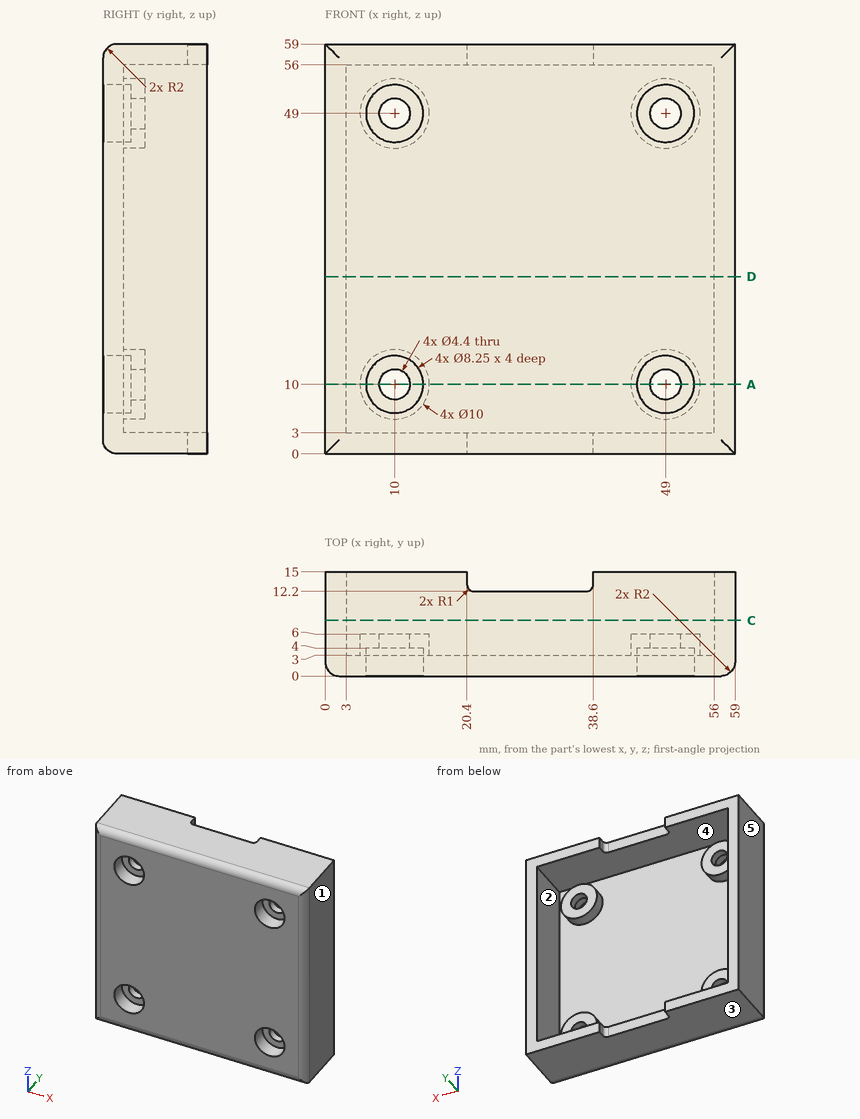
Can you work these out from the drawing? Everything is in mm from the part's minimum corner. A direction names the side the tool comes from. Round coordinates to 2 decimals unless told otherwise and drop trailing zeros. Order: outer loops, then holes, each group sorted by start corner. A loop starts at its lowest first (then second) coordinate and runs counter-clockwise, first axis right, second up. Notation, with made-up numbers: M 86,-9.5 L 132,-9.5 A20 ccw 132,5.5 Z; hole C -1,25 d11. An arc over 180 degrees is marked long. One line per question, with ' | ' between items.
1) For the marked faces 1 and 2, which set-ups out of +Z, -Z, +X, -X, +Y, -Y let a thin tool reach every point of the face, with its end or its side?
Working result:
face 1: +Z, -Z, +X, +Y, -Y | face 2: +Y
2) If we mould it in two halves opening along Z, with no side actions, what happens to the marked faces 3, 4 and 5? For each: +Z half, -Z half, draft (parallel to the pull), parting line (faces both ways), or undercut.
Working result:
face 3: -Z half | face 4: undercut | face 5: draft
3) I want a section at D-D, the plane z = 25.5. Write out the boundary of the cut face in (x, y), then the cut area to 3 significant figures.
Working result:
outline: M 0,2 A2 ccw 2,0 L 57,0 A2 ccw 59,2 L 59,15 L 56,15 L 56,3 L 3,3 L 3,15 L 0,15 Z | area: 247 mm²
4) I want a section at C-C, the plane y = 8. Write out the boundary of the cut face in (x, z).
Working result:
outline: M 0,0 L 59,0 L 59,59 L 0,59 Z; hole M 3,3 L 56,3 L 56,56 L 3,56 Z
5) I need wall thicknesses on line 1 along Z through (x, y) = (49, 5.3); line 2 along Z through (x, y) = (42, 14); line 3 along Z through (x, y) = (49, 2.3) (3 decimals). Which ranges of each line are inside material? Lowest first, please.
Working result:
line 1: 0 to 3, 5 to 7.8, 12.2 to 15, 44 to 46.8, 51.2 to 54, 56 to 59 | line 2: 0 to 3, 56 to 59 | line 3: 0 to 5.875, 14.125 to 44.875, 53.125 to 59
6) I want a section at A-A, the plane z = 10. State how many separate pieces and enclosed holes the cut face has, then the cut area to 3 significant figures.
Working result:
separate pieces: 3 | enclosed holes: 0 | area: 224 mm²
7) For pin 1 Ø5 at (x, z) = (23, 49) entering from +Y; pin 2 Ø4 at (x, z) = (49, 10) entering from +Y; pin 3 Ø5 at (x, z) = (49, 49) entering from +Y; pin 4 Ø3.5 at (x, z) = (28.5, 57) entering from +Y, each with a flat end and sliding along its axis, tell me the tip position at first contact or that it passes through.
Working result:
pin 1: y = 3 | pin 2: through | pin 3: y = 6 | pin 4: y = 12.2
